Design review of the part built by this model. Coordinates are the model's own, in mm. A direction names the side the tool comes from. Round coordinates to 2 decimals unless told otherwise and drop trailing zeros. Loops run counter-clockwise (first coordinate to the right, second up) from the corner with the lowest first, then second, coordinate; pieces in that order, holes last. Notation, with made-up numbers: (46.5, 7) -> (53.5, 7) arc R14 cw to (53.5, 14) -> close; hole circle Ø3 at (-28, 15). An arc over 180 degrees is marked (long way). Use a Markdown table: item, result. Add a question column.
from build123d import *

# Parameters (mm, degrees)
BOSS_EXTRUDE1_DEPTH = 38.1
CUT_EXTRUDE10_DEPTH = 7.62
SHELL2_START        = 6.35
SHELL2_DEPTH        = 31.75
SHELL2_2_DEPTH      = 17.78


# Read off the part's stored shape, not the designer's step: Shell2
with BuildPart() as part:
    # Sketch1 → Boss-Extrude1 (new body)
    with BuildSketch(Plane(origin=(0, 0, 0), x_dir=(1, 0, 0), z_dir=(0, 1, 0))):
        with BuildLine():
            Line((0, 11.43), (0, -11.43))
            Line((0, -11.43), (35.052, -5.249386672))
            Line((35.052, -5.249386672), (35.052, -19.981386672))
            Line((35.052, -19.981386672), (136.652, -19.981386672))
            Line((136.652, -19.981386672), (136.652, -70.781386672))
            ThreePointArc((136.652, -70.781386672), (154.559, -88.688386672), (172.466, -70.781386672))
            Line((172.466, -70.781386672), (172.466, 70.781386672))
            ThreePointArc((172.466, 70.781386672), (154.559, 88.688386672), (136.652, 70.781386672))
            Line((136.652, 70.781386672), (136.652, 19.981386672))
            Line((136.652, 19.981386672), (35.052, 19.981386672))
            Line((35.052, 19.981386672), (35.052, 5.249386672))
            Line((35.052, 5.249386672), (0, 11.43))
        make_face()
    extrude(amount=BOSS_EXTRUDE1_DEPTH)

    # Sketch5 → Cut-Extrude10 (cut)
    with BuildSketch(Plane(origin=(0, 38.1, 0), x_dir=(1, 0, 0), z_dir=(0, 1, 0))):
        Polygon((0, -11.43), (0, 11.43), (0.210478784, 11.603037745), (35.052, 5.249386672), (35.052, -5.249386672), align=None)
    extrude(amount=-CUT_EXTRUDE10_DEPTH, mode=Mode.SUBTRACT)

    # Shell2 outline → Shell2 (cut)
    with BuildSketch(Plane(origin=(0, 0, 0), x_dir=(1, 0, 0), z_dir=(0, 1, 0)).offset(SHELL2_START)):
        with BuildLine():
            Line((41.402, 13.631386672), (41.402, -13.631386672))
            Line((41.402, -13.631386672), (143.002, -13.631386672))
            Line((143.002, -13.631386672), (143.002, -70.781386672))
            ThreePointArc((143.002, -70.781386672), (154.559, -82.338386672), (166.116, -70.781386672))
            Line((166.116, -70.781386672), (166.116, 70.781386672))
            ThreePointArc((166.116, 70.781386672), (154.559, 82.338386672), (143.002, 70.781386672))
            Line((143.002, 70.781386672), (143.002, 13.631386672))
            Line((143.002, 13.631386672), (41.402, 13.631386672))
        make_face()
    extrude(amount=SHELL2_DEPTH, mode=Mode.SUBTRACT)

    # Shell2 2 outline → Shell2 2 (cut)
    with BuildSketch(Plane(origin=(0, 0, 0), x_dir=(1, 0, 0), z_dir=(0, 1, 0)).offset(SHELL2_START)):
        Polygon((28.25455863, 0), (6.35, 3.862364687), (6.35, -3.862364687), align=None)
    extrude(amount=SHELL2_2_DEPTH, mode=Mode.SUBTRACT)


solid = part.part
1. Consider section B-B on y = 28. State the section outline as (x, z) points.
2. For faces 1 (the face through (17.281, 15.027, 8.383)), 2 (the face through (91, 22, 13.631)), 3 (the face through (17.456, 15.116, -1.904)), list the 3-axis set-ups (+Z, -Z, +X, -X, +Y, -Y) from which the entire face can be reached by the end or side of a thin tool; tool diameter is ignored.
3. Consider section A-A on y = 15. State the section outline as (x, z) points.
4. Insertion check: P1, Ø5, axis at y = 30, z = -20, coming from the -X side; P2, Ø9.5, axis at x = 91, y = 21, coming from the +Z side; P3, Ø1, axis at y = 32, z = -59.5, coming from the -X side. Each pin has a flat end and moves straight along its axis. Give the tip position at first contact, or say it passes through.
5. Consider section C-C on x = 76. State the section outline as (y, z) points, plus the area to 3 significant figures.
6. Consider section D-D on z = 48. State the section outline as (x, y) points.
7. To check wall thickness, follow probe 1 along X at (y, z) = (20, 63.5); probe 2 along Y at (x, z) = (153, -67.5); probe 3 along Z at (x, y) = (132, 33). State the ranges of each line that lie inside material, in increasing order. Write a range as from..to.
8. Mouldability with a two-part tool opening along X and no side actions: class faces 4 (the face through (85, 19, 19.981)), 5 (the face through (17.771, 15.027, -8.296)), 6 (the face through (136.652, 19, -46)) as +X half, -X half, draft (parallel to the pull), parting line (faces both ways), or undercut.
Verdict:
| question | item | result |
|---|---|---|
| 1 | outline | (0, -11.43) -> (35.05, -5.25) -> (35.05, -19.98) -> (136.65, -19.98) -> (136.65, -70.78) arc R17.91 ccw to (172.47, -70.78) -> (172.47, 70.78) arc R17.91 ccw to (136.65, 70.78) -> (136.65, 19.98) -> (35.05, 19.98) -> (35.05, 5.25) -> (0, 11.43) -> close; hole (41.4, -13.63) -> (143, -13.63) -> (143, -70.78) arc R11.56 ccw to (166.12, -70.78) -> (166.12, 70.78) arc R11.56 ccw to (143, 70.78) -> (143, 13.63) -> (41.4, 13.63) -> close |
| 2 | face 1 | +Z, +Y, -Y |
| 2 | face 2 | +Y |
| 2 | face 3 | none |
| 3 | outline | (0, -11.43) -> (35.05, -5.25) -> (35.05, -19.98) -> (136.65, -19.98) -> (136.65, -70.78) arc R17.91 ccw to (172.47, -70.78) -> (172.47, 70.78) arc R17.91 ccw to (136.65, 70.78) -> (136.65, 19.98) -> (35.05, 19.98) -> (35.05, 5.25) -> (0, 11.43) -> close; hole (6.35, -3.86) -> (28.25, 0) -> (6.35, 3.86) -> close; hole (41.4, -13.63) -> (143, -13.63) -> (143, -70.78) arc R11.56 ccw to (166.12, -70.78) -> (166.12, 70.78) arc R11.56 ccw to (143, 70.78) -> (143, 13.63) -> (41.4, 13.63) -> close |
| 4 | P1 | stops at x = 35.05 |
| 4 | P2 | stops at z = 19.98 |
| 4 | P3 | stops at x = 136.65 |
| 5 | outline | (0, -19.98) -> (38.1, -19.98) -> (38.1, -13.63) -> (6.35, -13.63) -> (6.35, 13.63) -> (38.1, 13.63) -> (38.1, 19.98) -> (0, 19.98) -> close |
| 5 | area | 657 mm² |
| 6 | outline | (136.65, 0) -> (172.47, 0) -> (172.47, 38.1) -> (166.12, 38.1) -> (166.12, 6.35) -> (143, 6.35) -> (143, 38.1) -> (136.65, 38.1) -> close |
| 7 | probe 1 | x = 136.65..143, 166.12..172.47 |
| 7 | probe 2 | y = 0..6.35 |
| 7 | probe 3 | z = -19.98..-13.63, 13.63..19.98 |
| 8 | face 4 | draft |
| 8 | face 5 | undercut |
| 8 | face 6 | -X half |
